For this review, use the dimensioned drawing (mm, ordinates from the lowest corner) and the shaded views. A direction names the side the tool comes from. Give positions to 0.01 mm unless a question says otherwise; leave off trailing zeros. Order: outer loops, then holes, each group sorted by start corner. A loop starts at its lowest first (then second) coordinate and runs counter-clockwise, first axis right, second up.
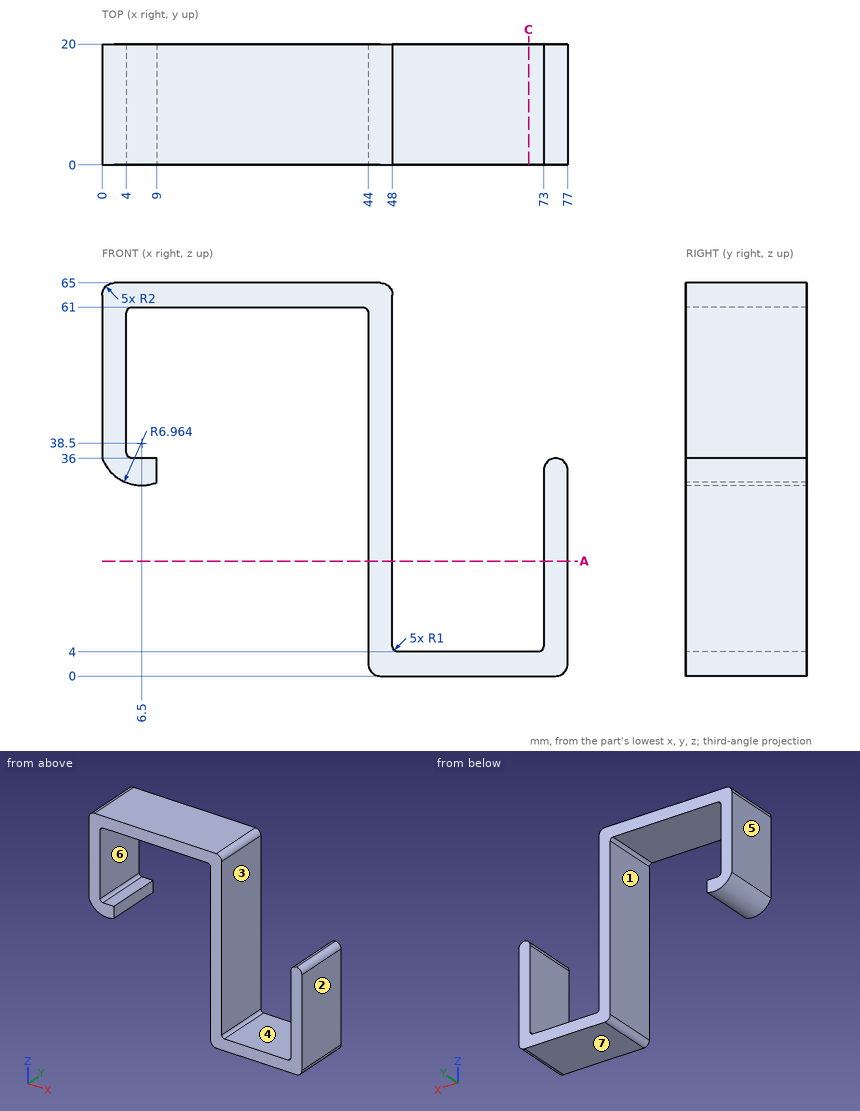
1. Take a section at A-A (z = 19). State the section outline as (x, y) points.
Recorded:
outline: (44, 0) - (48, 0) - (48, 20) - (44, 20) - close; (73, 0) - (77, 0) - (77, 20) - (73, 20) - close
2. Machinability: for the marked faces 1, 2 and 3, which of the approach directions +Z, -Z, +X, -X, +Y, -Y give a long, thin tool a straight path to every point of the face, cutting with its end or side? Answer none if there is none.
Recorded:
face 1: -Z, +Y, -Y
face 2: +Z, -Z, +X, +Y, -Y
face 3: +Z, +Y, -Y
3. Take a section at C-C (x = 70.5). State the section outline as (y, z) points.
Recorded:
outline: (0, 0) - (20, 0) - (20, 4) - (0, 4) - close
4. Draft analysis for pull direction Z (two halves, no side actions). For the marked faces 4, 5, 6 and 7, state which applies: pulls with the +Z half, pulls with the -Z half, needs draft (parallel to the pull), parting line crosses it, or undercut.
Recorded:
face 4: pulls with the +Z half
face 5: needs draft
face 6: undercut
face 7: pulls with the -Z half
5. For pin 1 (6 mm diameter, centred on y = 3.5, z = 50.5, fed in from +X); pin 2 (3 mm diameter, centred on y = 8.5, z = 35, fed in from +X); pin 3 (6 mm diameter, centred on x = 15, y = 13.5, fed in from -Z), all flat-tipped, find the tip position at first contact; note any pin that passes through.
Recorded:
pin 1: stops at x = 48
pin 2: stops at x = 77
pin 3: stops at z = 61
6. For line 1 along X through (y, z) = (1.75, 17); line 2 along X through (y, z) = (8.25, 54.5); line 3 along Z through (x, y) = (7, 10), list the stretches that pass through material, from the lowest coordinate up.
Recorded:
line 1: x = 44 to 48, 73 to 77
line 2: x = 0 to 4, 44 to 48
line 3: z = 31.55 to 36, 61 to 65
